Here's how the part is built. I have some questions about the finished solid (model axes, mm). Face numbers are marked on the shaded views. A direction names the side the tool comes from. Coordinates: 2 decimals unless noted, no trailing zeros. Loops run counter-clockwise (first coordinate to the right, second up) from the corner with the lowest first, then second, coordinate; pieces in that order, holes last. Notation, with made-up numbers: (-26, 80) - (16, 80) arc R12 cw to (16, 91) - close; hole circle Ø11 at (0.25, 14.5). An arc over 180 degrees is marked (long way). Use a Markdown table: item, result.
Autodesk Inventor part; units mm, degrees
ref_plane "YZ Plane" through (0, 0, 0) normal (1, 0, 0) x (0, 1, 0)
ref_plane "XZ Plane" through (0, 0, 0) normal (0, 1, 0) x (-1, 0, 0)
ref_plane "XY Plane" through (0, 0, 0) normal (0, 0, 1) x (1, 0, 0)
sketch "Sketch1" plane through (0, 0, 0) normal (0, 0, 1) x (1, 0, 0)
  line L0 (0, 67.3) -> (0, 0)
  line L1 (0, 0) -> (60, 0)
  line L2 (60, 0) -> (60, 16)
  line L3 (60, 16) -> (8, 67.3)
  line L4 (8, 67.3) -> (0, 67.3)
  dimension "d0" = 67.3
  dimension "d1" = 8
  dimension "d2" = 16
  dimension "d3" = 60
extrude "Extrusion1" add sketch "Sketch1" along normal blind 6.5
sketch "Sketch2" plane through (0, 0, 6.5) normal (0, 0, 1) x (1, 0, 0)
  line L0 (0, 67.3) -> (0, 0)
  line L1 (0, 0) -> (60, 0)
  line L2 (60, 0) -> (60, 16)
  line L3 (8, 67.3) -> (0, 67.3)
  line L4 (16.3, 50.05) -> (16.3, 45.55)
  line L5 (0, 45.55) -> (0, 50.05)
  line L6 (5, 52.55) -> (12.3, 52.55)
  line L7 (12.3, 43.05) -> (5, 43.05)
  line L8 (38.25, 16.3) -> (42.75, 16.3)
  line L9 (42.75, 0) -> (38.25, 0)
  line L10 (45.25, 12.3) -> (45.25, 5)
  line L11 (35.75, 5) -> (35.75, 12.3)
  line L12 (5, 43.05) -> (5, 45.55)
  line L13 (5, 50.05) -> (5, 52.55)
  line L14 (12.3, 52.55) -> (12.3, 50.05)
  line L15 (12.3, 45.55) -> (12.3, 43.05)
  line L16 (0, 50.05) -> (5, 50.05)
  line L17 (12.3, 50.05) -> (16.3, 50.05)
  line L18 (16.3, 45.55) -> (12.3, 45.55)
  line L19 (5, 45.55) -> (0, 45.55)
  line L20 (35.75, 12.3) -> (38.25, 12.3)
  line L21 (42.75, 12.3) -> (45.25, 12.3)
  line L22 (45.25, 5) -> (42.75, 5)
  line L23 (38.25, 5) -> (35.75, 5)
  line L24 (38.25, 0) -> (38.25, 5)
  line L25 (38.25, 12.3) -> (38.25, 16.3)
  line L26 (42.75, 16.3) -> (42.75, 12.3)
  line L27 (42.75, 5) -> (42.75, 0)
  point P0 (16.3, 47.8)
  point P1 (40.5, 16.3)
  dimension "d6" = 4.5
  dimension "d7" = 5
  dimension "d8" = 7.3
  dimension "d9" = 4
  dimension "d10" = 2.5
  dimension "d11" = 19.5
  dimension "d12" = 19.5
extrude "Extrusion2" cut sketch "Sketch2" against normal through all
sketch "Sketch3" plane through (0, 0, 6.5) normal (0, 0, 1) x (1, 0, 0)
  line L0 (0, 45.55) -> (0, 0)
  line L1 (0, 0) -> (38.25, 0)
  line L2 (38.25, 16.3) -> (42.75, 16.3)
  line L3 (42.75, 0) -> (60, 0)
  line L4 (0, 67.3) -> (0, 50.05)
  line L5 (16.3, 50.05) -> (16.3, 45.55)
  line L6 (0, 40.3) -> (-4.5, 40.3)
  line L7 (-6.5, 38.3) -> (-6.5, 34.3)
  line L8 (-4.5, 32.3) -> (0, 32.3)
  line L9 (0, 32.3) -> (0, 40.3)
  line L10 (0, 63.3) -> (-4.5, 63.3)
  line L11 (-6.5, 61.3) -> (-6.5, 57.3)
  line L12 (-4.5, 55.3) -> (0, 55.3)
  line L13 (0, 55.3) -> (0, 63.3)
  line L14 (25, 0) -> (33, 0)
  line L15 (33, 0) -> (33, -4.5)
  line L16 (31, -6.5) -> (27, -6.5)
  line L17 (25, -4.5) -> (25, 0)
  line L18 (48, 0) -> (56, 0)
  line L19 (56, 0) -> (56, -4.5)
  line L20 (54, -6.5) -> (50, -6.5)
  line L21 (48, -4.5) -> (48, 0)
  arc A0 (-4.5, 63.3) -> (-6.5, 61.3) centre (-4.5, 61.3) ccw
  arc A1 (-6.5, 57.3) -> (-4.5, 55.3) centre (-4.5, 57.3) ccw
  arc A2 (-4.5, 40.3) -> (-6.5, 38.3) centre (-4.5, 38.3) ccw
  arc A3 (-6.5, 34.3) -> (-4.5, 32.3) centre (-4.5, 34.3) ccw
  arc A4 (25, -4.5) -> (27, -6.5) centre (27, -4.5) ccw
  arc A5 (31, -6.5) -> (33, -4.5) centre (31, -4.5) ccw
  arc A6 (48, -4.5) -> (50, -6.5) centre (50, -4.5) ccw
  arc A7 (54, -6.5) -> (56, -4.5) centre (54, -4.5) ccw
  point P0 (16.3, 47.8)
  point P1 (40.5, 16.3)
  dimension "d15" = 2
  dimension "d16" = 8
  dimension "d17" = 8
  dimension "d18" = 8
  dimension "d19" = 8
  dimension "d20" = 6.5
  dimension "d21" = 6.5
  dimension "d22" = 15
  dimension "d23" = 15
  dimension "d24" = 7.5
  dimension "d25" = 7.5
extrude "Extrusion3" add sketch "Sketch3" against normal blind 6.5
equation "\"d21\" = d20"
properties part number "y_motor_mount_brace" material "Plywood, Finish"
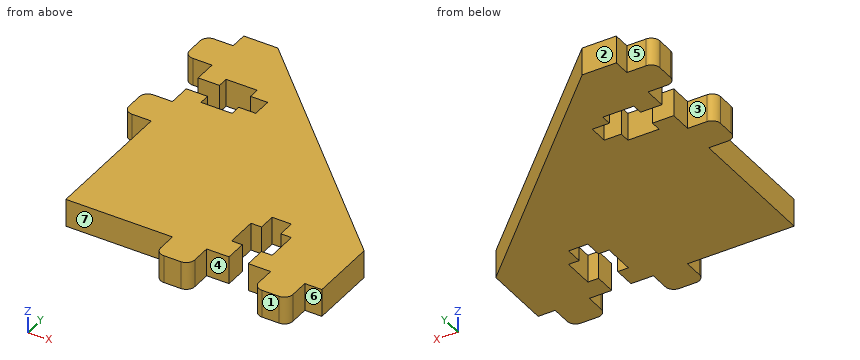
Q1. I want a section at A-A, the plane y = 15. Write out the boundary of the cut face in (x, z).
Check values:
| item | result |
|---|---|
| outline | (0, 0) - (38.25, 0) - (38.25, 6.5) - (0, 6.5) - close; (42.75, 0) - (60, 0) - (60, 6.5) - (42.75, 6.5) - close |
Q2. Which directions (+Z, -Z, +X, -X, +Y, -Y) give clear straight access to the entire face, cutting with the end or side of a thin tool? Please do the marked faces 4, 5, 6 and 7.
Check values:
| item | result |
|---|---|
| face 4 | +Z, -Z, -Y |
| face 5 | +Z, -Z, -X, +Y |
| face 6 | +Z, -Z, +X, -Y |
| face 7 | +Z, -Z, -X, -Y |
Q3. I want a section at B-B, the plane x = 14. Write out the boundary of the cut face in (y, z), then the cut area to 3 significant figures.
Check values:
| item | result |
|---|---|
| outline | (0, 0) - (45.55, 0) - (45.55, 6.5) - (0, 6.5) - close; (50.05, 0) - (61.38, 0) - (61.38, 6.5) - (50.05, 6.5) - close |
| area | 370 mm^2 |
Q4. I want a section at C-C, the plane x = 41.5. Write out the boundary of the cut face in (y, z).
Check values:
| item | result |
|---|---|
| outline | (16.3, 0) - (34.25, 0) - (34.25, 6.5) - (16.3, 6.5) - close |
Q5. Will these pins go through, and if not, where does the flat tip stop? P1, Ø2, axis at y = 16.5, z = 2, coming from the -X side; P2, Ø1.3, axis at x = -1.5, z = 3.5, coming from the +Y side; P3, Ø3, axis at x = 52, y = 5, coming from the -Z side; P4, Ø3, axis at x = 37.5, z = 4, coming from the -Y side.
Check values:
| item | result |
|---|---|
| P1 | x = 0 |
| P2 | y = 63.3 |
| P3 | z = 0 |
| P4 | y = 0 |
Q6. I want a section at D-D, the plane x = 34.5. Write out the boundary of the cut face in (y, z).
Check values:
| item | result |
|---|---|
| outline | (0, 0) - (41.16, 0) - (41.16, 6.5) - (0, 6.5) - close |
Q7. Please list where these lines run through material, in increasing order: L1, parallel to X at y = 3, z = 1; L2, parallel to X at y = 6, z = 1.5; L3, parallel to Y at x = 8.5, z = 2.5. Write a range as from..to.
Check values:
| item | result |
|---|---|
| L1 | 0..38.25, 42.75..60 |
| L2 | 0..35.75, 45.25..60 |
| L3 | 0..43.05, 52.55..66.81 |
Q8. If we mould it in two halves opening along Y, with no side actions, what happens to the marked faces 1, 2 and 3? For each: pulls with the +Y half, pulls with the -Y half, needs draft (parallel to the pull), parting line crosses it, or undercut.
Check values:
| item | result |
|---|---|
| face 1 | pulls with the -Y half |
| face 2 | pulls with the +Y half |
| face 3 | undercut |
